Model file for the job. Use its own axes, mm. Face numbers are marked on the shaded views. A direction names the side the tool comes from. Give positions to 0.01 mm unless a question says otherwise; leave off trailing zeros. Order: outer loops, then holes, each group sorted by start corner. A loop starts at its lowest first (then second) coordinate and runs counter-clockwise, first axis right, second up. Notation, with made-up numbers: M 15.5,41 L 45.5,41 A19 ccw 45.5,48 Z; hole C 88,36 d3. An arc over 180 degrees is marked long. Return JSON: item names as keys, results as strings. Group by question number.
1. Slice it at D-D on z = -21. List the corners of the cut face in (x, y) (3 decimals), then the cut area to 3 significant figures.
2. Pin check, flat tips, straight feed: pin 1 (3 mm diameter, centred on x = 16.5, y = 119.5, fed in from +Z); pin 2 (1.5 mm diameter, centred on x = -2.5, y = 37.5, fed in from +Z); pin 3 (2 mm diameter, centred on y = 77.5, z = -1, fed in from +X). Stop position of each tip, or through.
3. Wall check: probe 1 along X at (y, z) = (126, -12); probe 2 along X at (y, z) = (0, 3) (3 decimals); probe 3 along Y at (x, z) = (0, 5.25) (3 decimals). Give the ranges that are in metal, low to high. Write a range as [from, to].
4. 3-axis set-ups, long thin cutter, end or side, ignore diameter. For the marked faces 5, 6 and 7: which of +Z, -Z, +X, -X, +Y, -Y reach the whole face in a straight line?
5. Two-plate mould, pull along X, no slides. Class the marked faces 1, 2, 3 and 4: released by +X, released by -X, zero draft, split by the parting line, or undercut.
6. Slice it at A-A on x = 0. List the corners of the cut face in (y, z) (3 decimals), then the cut area to 3 significant figures.
7. Slice it at C-C on y = 75.5. List the corners of the cut face in (x, z).
8. Slice it at B-B on y = 0. List the corners of the cut face in (x, z) (3 decimals).
from build123d import *
from build123d.topology import SkipClean

# Parameters (mm, degrees)
SKETCH1_R            = 28.574999999999996
BASE_PIVOT_DEPTH     = 12.7
SHAFT_START          = -12.7
SHAFT_DEPTH          = 12.7
TOP_START            = 1.524
SKETCH3_R            = 21.335999999999974
TOP_SHELF_DEPTH      = 1.524
SKETCH4_R            = 12.699999999999998
TOP_PIN_DEPTH        = 50.8
FRONT_START          = -2.54
FRONT_RECESS_DEPTH   = 2.54
BACK_RECESS_DEPTH    = 2.54
BASE_HOLE_DEPTH      = 209.43551693989195
BASE_HOLE_DEPTH_BACK = 209.43551693989195
SKETCH7_R            = 12.7
KEY_WAY_DEPTH        = 209.43551693989195
KEY_WAY_DEPTH_BACK   = 209.43551693989195
FILLET1_R            = 3.175


with BuildPart() as part:
    # Sketch1 → Base pivot (new, symmetric)
    with BuildSketch(Plane.XY):
        Circle(SKETCH1_R)
    extrude(amount=BASE_PIVOT_DEPTH, both=True)

    # Sketch2 → Shaft (add)
    with BuildSketch(Plane.XY.offset(SHAFT_START)):
        with BuildLine():
            Line((-21.335999999999938, 174.625), (-21.336000000000002, 7.84e-15))
            Line((-21.336000000000002, 7.84e-15), (21.336000000000002, 0))
            Line((21.336000000000002, 0), (21.336000000000002, 174.625))
            ThreePointArc((21.336000000000002, 174.625), (3.338e-14, 195.96099999999996), (-21.335999999999938, 174.625))
        make_face()
    extrude(amount=SHAFT_DEPTH)

    # Sketch3 → Top shelf (add)
    with SkipClean():  # the faces are left unmerged after this step: merging them gives an invalid solid
        with BuildSketch(Plane(origin=(0, 0, -12.7), x_dir=(-1, 0, 0), z_dir=(0, 0, -1)).offset(TOP_START)):
            with Locations((-3.208e-14, 174.625)):
                Circle(SKETCH3_R)
        extrude(amount=-TOP_SHELF_DEPTH)

    # Sketch4 → Top pin (add)
    with SkipClean():  # the faces are left unmerged after this step: merging them gives an invalid solid
        with BuildSketch(Plane(origin=(0, 0, -14.223999999999998), x_dir=(-1, 0, 0), z_dir=(0, 0, -1))):
            with Locations((-3.208e-14, 174.625)):
                Circle(SKETCH4_R)
        extrude(amount=TOP_PIN_DEPTH)

    # Sketch5 → Front recess (cut)
    with SkipClean():  # the faces are left unmerged after this step: merging them gives an invalid solid
        with BuildSketch(Plane.XY.offset(FRONT_START)):
            with BuildLine():
                Line((-13.461999999999927, 158.07207119570683), (-13.461999999999975, 25.20526097861318))
                ThreePointArc((-13.461999999999975, 25.20526097861318), (1.75e-15, 28.574999999999992), (13.461999999999987, 25.205260978613172))
                Line((13.461999999999987, 25.205260978613172), (13.462000000000003, 158.07207119570683))
                ThreePointArc((13.462000000000003, 158.07207119570683), (3.812e-14, 153.28900000000004), (-13.461999999999927, 158.07207119570683))
            make_face()
        extrude(amount=FRONT_RECESS_DEPTH, mode=Mode.SUBTRACT)

    # Sketch6 → Back recess (cut)
    with SkipClean():  # the faces are left unmerged after this step: merging them gives an invalid solid
        with BuildSketch(Plane(origin=(0, 0, -12.7), x_dir=(-1, 0, 0), z_dir=(0, 0, -1))):
            with BuildLine():
                Line((13.461999999999929, 158.07207119570683), (13.461999999999975, 25.20526097861318))
                ThreePointArc((13.461999999999975, 25.20526097861318), (-1.094e-14, 28.574999999999992), (-13.461999999999987, 25.205260978613172))
                Line((-13.461999999999987, 25.205260978613172), (-13.461999999999998, 158.07207119570683))
                ThreePointArc((-13.461999999999998, 158.07207119570683), (-3.551e-14, 153.28900000000004), (13.461999999999929, 158.07207119570683))
            make_face()
        extrude(amount=-BACK_RECESS_DEPTH, mode=Mode.SUBTRACT)

    # Sketch7 → Base hole (cut, two sides: drawn at the far end of the back side and taken through both)
    with SkipClean():  # the faces are left unmerged after this step: merging them gives an invalid solid
        with BuildSketch(Plane.XY.offset(-BASE_HOLE_DEPTH_BACK)):
            Circle(SKETCH7_R)
        extrude(amount=BASE_HOLE_DEPTH + BASE_HOLE_DEPTH_BACK, mode=Mode.SUBTRACT)

    # Sketch8 → Key way (cut, two sides: drawn at the far end of the back side and taken through both)
    with SkipClean():  # the faces are left unmerged after this step: merging them gives an invalid solid
        with BuildSketch(Plane.XY.offset(-KEY_WAY_DEPTH_BACK)):
            Polygon((4e-16, 3.1750000000000003), (15.875, 3.174999999999997), (15.875, -3.1750000000000034), (-7.7e-16, -3.1750000000000003), align=None)
        extrude(amount=KEY_WAY_DEPTH + KEY_WAY_DEPTH_BACK, mode=Mode.SUBTRACT)

    # Fillet1
    # the kernel refuses this fillet: 3.175 mm, written as the material it adds along each edge
    with BuildSketch(Plane(origin=(-13.461999999999927, 158.07207119570683, -16.77729862803093), x_dir=(0.8483467712248999, -0.5294409842015325, 0), z_dir=(0, 0, 1))) as fillet1_piece_1_section:
        with BuildLine():
            CenterArc((5.70862475783739, -3.1502914039819587), FILLET1_R, 97.15273031823853, 114.81496184230716)
            Line((3.0151237591983637, -4.831266528821872), (0, 0))
            ThreePointArc((0, 0), (2.656645316666723, -0.16604176524117806), (5.313290633333425, -6e-17))
        make_face()
    fillet1_piece_1 = extrude(amount=16.77729862803093, mode=Mode.PRIVATE)
    fillet1_piece_1 = split(fillet1_piece_1, bisect_by=Plane(origin=(-12.378027921631585, 155.86897654595924, -12.7), z_dir=(0, 0, 1)), keep=Keep.TOP, mode=Mode.PRIVATE)
    add(fillet1_piece_1)
    with BuildSketch(Plane(origin=(13.462000000000003, 158.07207119570683, -16.777298628030998), x_dir=(0, -1, 0), z_dir=(0, 0, 1))) as fillet1_piece_2_section:
        with BuildLine():
            CenterArc((5.6949194512123995, -3.1750000000000007), FILLET1_R, 90, 114.81496184230605)
            ThreePointArc((2.813073822260918, -4.50751295336787), (1.5473979065612582, -2.1658471610760905), (0, 0))
            Line((0, 0), (5.6949194512123995, 0))
        make_face()
    fillet1_piece_2 = extrude(amount=16.777298628030998, mode=Mode.PRIVATE)
    fillet1_piece_2 = split(fillet1_piece_2, bisect_by=Plane(origin=(12.378027921631652, 155.86897654595924, -12.7), z_dir=(0, 0, 1)), keep=Keep.TOP, mode=Mode.PRIVATE)
    add(fillet1_piece_2)
    with BuildSketch(Plane(origin=(13.461999999999982, 25.205260978613172, -14.620128336437258), x_dir=(-0.9170202383773097, 0.39884067295904263, 0), z_dir=(0, 0, 1))) as fillet1_piece_3_section:
        with BuildLine():
            CenterArc((4.838757862902442, -3.1647697300383113), FILLET1_R, 94.60072202830712, 108.90500130287109)
            Line((1.9272186060544878, -4.431088866683278), (0, 0))
            ThreePointArc((0, 0), (2.2920431982169482, -0.0920724296552107), (4.584086396433892, 1.4e-16))
        make_face()
    fillet1_piece_3 = extrude(amount=14.620128336437258, mode=Mode.PRIVATE)
    fillet1_piece_3 = split(fillet1_piece_3, bisect_by=Plane(origin=(12.464896317702909, 26.864585865403097, -12.7), z_dir=(0, 0, 1)), keep=Keep.TOP, mode=Mode.PRIVATE)
    add(fillet1_piece_3)
    with BuildSketch(Plane(origin=(-13.461999999999975, 25.20526097861318, -14.620128336437222), x_dir=(0.9170202383773097, 0.3988406729590427, 0), z_dir=(0, 0, 1))) as fillet1_piece_4_section:
        with BuildLine():
            CenterArc((4.838757862902452, 3.164769730038311), FILLET1_R, 156.49427666882212, 108.90500130287074)
            Line((1.927218606054489, 4.431088866683262), (0, 0))
            ThreePointArc((0, 0), (2.292043198216952, 0.09207242965520915), (4.5840863964339, 1e-17))
        make_face()
    fillet1_piece_4 = extrude(amount=14.620128336437222, mode=Mode.PRIVATE)
    fillet1_piece_4 = split(fillet1_piece_4, bisect_by=Plane(origin=(-12.464896317702895, 26.864585865403104, -12.7), z_dir=(0, 0, 1)), keep=Keep.TOP, mode=Mode.PRIVATE)
    add(fillet1_piece_4)
    with BuildSketch(Plane(origin=(13.462, 158.07207119570683, -12.7), x_dir=(0, -1, 0), z_dir=(0, 0, 1))) as fillet1_piece_5_section:
        with BuildLine():
            CenterArc((5.6949194512123995, -3.1750000000000007), FILLET1_R, 90, 114.81496184230605)
            ThreePointArc((2.813073822260918, -4.50751295336787), (1.5473979065612582, -2.1658471610760905), (0, 0))
            Line((0, 0), (5.6949194512123995, 0))
        make_face()
    fillet1_piece_5 = extrude(amount=16.777298628031005, mode=Mode.PRIVATE)
    fillet1_piece_5 = split(fillet1_piece_5, bisect_by=Plane(origin=(12.378027921631652, 155.86897654595924, 0), z_dir=(0, 0, -1)), keep=Keep.TOP, mode=Mode.PRIVATE)
    add(fillet1_piece_5)
    with BuildSketch(Plane(origin=(-13.46199999999993, 158.07207119570683, -12.7), x_dir=(-3.1e-16, -1, 0), z_dir=(0, 0, 1))) as fillet1_piece_6_section:
        with BuildLine():
            CenterArc((5.6949194512124555, 3.1750000000000007), FILLET1_R, 155.18503815769455, 114.81496184230548)
            ThreePointArc((2.8130738222609453, 4.507512953367848), (1.5473979065612575, 2.1658471610760963), (0, 0))
            Line((0, 0), (5.694919451212456, 0))
        make_face()
    fillet1_piece_6 = extrude(amount=16.777298628031147, mode=Mode.PRIVATE)
    fillet1_piece_6 = split(fillet1_piece_6, bisect_by=Plane(origin=(-12.378027921631558, 155.86897654595919, 0), z_dir=(0, 0, -1)), keep=Keep.TOP, mode=Mode.PRIVATE)
    add(fillet1_piece_6)
    with BuildSketch(Plane(origin=(-13.461999999999975, 25.20526097861318, -12.7), x_dir=(0, 1, 0), z_dir=(0, 0, 1))) as fillet1_piece_7_section:
        with BuildLine():
            CenterArc((4.832051334574889, -3.1750000000000007), FILLET1_R, 90, 108.905001302871)
            ThreePointArc((1.8283201032560825, -4.203700000000001), (0.9985923330184399, -2.0651277701953425), (0, 0))
            Line((0, 0), (4.832051334574889, 0))
        make_face()
    fillet1_piece_7 = extrude(amount=14.620128336437226, mode=Mode.PRIVATE)
    fillet1_piece_7 = split(fillet1_piece_7, bisect_by=Plane(origin=(-12.4648963177029, 26.8645858654031, 0), z_dir=(0, 0, -1)), keep=Keep.TOP, mode=Mode.PRIVATE)
    add(fillet1_piece_7)
    with BuildSketch(Plane(origin=(13.46199999999999, 25.205260978613172, -12.7), x_dir=(-0.9170202383773102, 0.3988406729590419, 0), z_dir=(0, 0, 1))) as fillet1_piece_8_section:
        with BuildLine():
            CenterArc((4.838757862902448, -3.164769730038312), FILLET1_R, 94.60072202830708, 108.905001302871)
            Line((1.927218606054491, -4.4310888666832735), (0, 0))
            ThreePointArc((0, 0), (2.2920431982169456, -0.09207242965520608), (4.584086396433901, -1e-17))
        make_face()
    fillet1_piece_8 = extrude(amount=14.620128336437253, mode=Mode.PRIVATE)
    fillet1_piece_8 = split(fillet1_piece_8, bisect_by=Plane(origin=(12.464896317702909, 26.8645858654031, 0), z_dir=(0, 0, -1)), keep=Keep.TOP, mode=Mode.PRIVATE)
    add(fillet1_piece_8)


solid = part.part
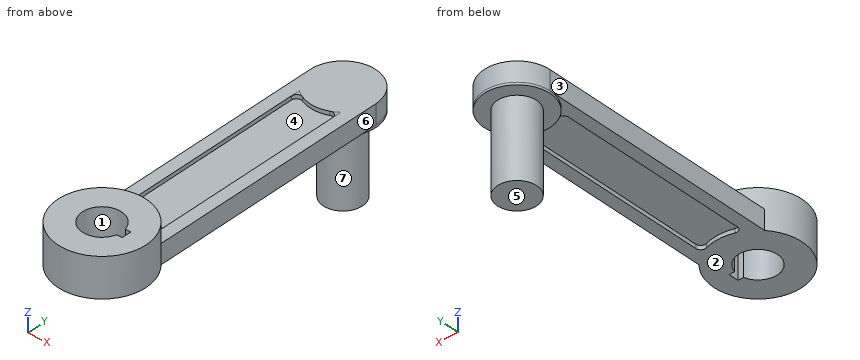
Result:
{
 "1": {"outline": "C 0,174.625 d25.4", "area": "507 mm2"},
 "2": {"pin 1": "stops at z = 0", "pin 2": "stops at z = -2.54", "pin 3": "stops at x = 21.34"},
 "3": {"probe 1": "x = [-21.34, -13.46], [13.46, 21.34]", "probe 2": "x = [-28.575, -12.7], [15.875, 28.575]", "probe 3": "y = [-28.575, -12.7], [12.7, 28.575]"},
 "4": {"face 5": "-Z, +X, -X, +Y, -Y", "face 6": "+Z, -Z, +X, +Y", "face 7": "-Z"},
 "5": {"face 1": "undercut", "face 2": "zero draft", "face 3": "released by -X", "face 4": "undercut"},
 "6": {"outline": "M -28.575,-12.7 L -12.7,-12.7 L -12.7,12.7 L -28.575,12.7 Z; M 12.7,-12.7 L 28.575,-12.7 L 28.575,-10.16 L 153.289,-10.16 L 153.289,-14.224 L 161.925,-14.224 L 161.925,-65.024 L 187.325,-65.024 L 187.325,-14.224 L 195.961,-14.224 L 195.961,0 L 153.289,0 L 153.289,-2.54 L 28.575,-2.54 L 28.575,12.7 L 12.7,12.7 Z", "area": "3,650 mm2"},
 "7": {"outline": "M -21.34,-12.7 L -13.46,-12.7 L -13.46,-10.16 L 13.46,-10.16 L 13.46,-12.7 L 21.34,-12.7 L 21.34,0 L 13.46,0 L 13.46,-2.54 L -13.46,-2.54 L -13.46,0 L -21.34,0 Z"},
 "8": {"outline": "M -28.575,-12.7 L -12.7,-12.7 L -12.7,12.7 L -28.575,12.7 Z; M 15.875,-12.7 L 28.575,-12.7 L 28.575,12.7 L 15.875,12.7 Z"}
}
